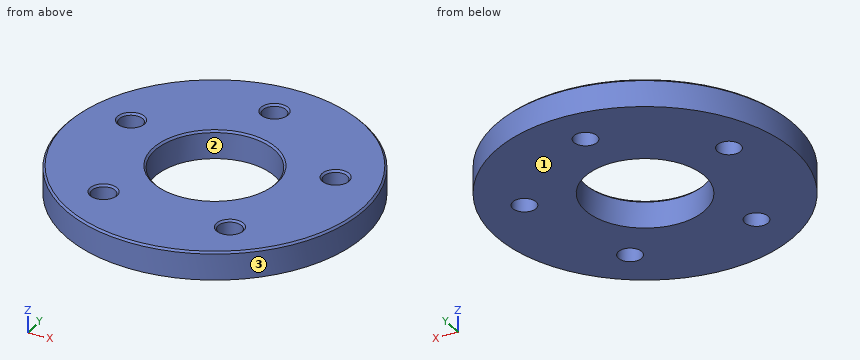
from build123d import *

# Parameters (mm, degrees)
F0_R     = 80
F0_R_2   = 6.25
F0_R_3   = 32.05
F1_DEPTH = 15
F2_SIZE  = 1


with BuildPart() as f1:
    # F0 (on Top) → F1 (new body)
    with BuildSketch(Plane.XY):
        Circle(F0_R)
        with Locations((-33.591927, -46.235321)):
            Circle(F0_R_2, mode=Mode.SUBTRACT)
        with Locations((33.591927, -46.235321)):
            Circle(F0_R_2, mode=Mode.SUBTRACT)
        with Locations((-54.35288, 17.660321)):
            Circle(F0_R_2, mode=Mode.SUBTRACT)
        Circle(F0_R_3, mode=Mode.SUBTRACT)
        with Locations((54.35288, 17.660321)):
            Circle(F0_R_2, mode=Mode.SUBTRACT)
        with Locations((0, 57.15)):
            Circle(F0_R_2, mode=Mode.SUBTRACT)
    extrude(amount=F1_DEPTH)

    # F2
    f2_edges = [f1.edges().sort_by_distance(p)[0] for p in [
        (-80, 0, 15),
        (-39.841927, -46.235321, 15),
        (27.341927, -46.235321, 15),
        (-60.60288, 17.660321, 15),
        (-32.05, 0, 15),
        (48.10288, 17.660321, 15),
        (-6.25, 57.15, 15),
    ]]
    chamfer(f2_edges, length=F2_SIZE)


solid = f1.part
Verification items for the finished model (mm, model axes). Face numbers are marked on the shaded views. Give positions to 0.01 mm unless a question says otherwise; leave off trailing zeros. Loops run counter-clockwise (first coordinate to the right, second up) from the corner with the lowest first, then second, coordinate; pieces in that order, holes last.
1) Sectioned sample at C-C, the plane z = 8.75. Enter the section's corners in (x, y), then the cut area to 3 significant figures.
2) Sectioned sample at B-B, the plane x = 0. Enter the section's corners in (y, z), then the cut area to 3 significant figures.
3) Thickness scan on line 1 along Y through (x, z) = (0, 4.5); line 2 along X through (y, z) = (0.5, 13.5); line 3 along X through (y, z) = (13.5, 12.5). Record the ranges inside material, lowest first.
4) Draft check along X on the marked faces 1, 2 and 3. Enter one of: pulls with the +X half, pulls with the -X half, needs draft (parallel to the pull), parting line crosses it, or undercut.
5) Depth check by flat-ended pin: pin 1 Ø3 at (y, z) = (6, 8) entering from +X; pin 2 Ø1 at (x, y) = (-44, 25) entering from -Z; pin 3 Ø2 at (y, z) = (26, 1.5) entering from +X; pin 4 Ø1.5 at (x, z) = (28.5, 5) entering from +Y. Enter the tip coordinate at first touch or a pass-through.
6) Sectioned sample at A-A, the plane y = 0. Enter the section's corners in (x, z).
Answers:
1. outline: circle Ø160 at (0, 0); hole circle Ø12.5 at (-54.35, 17.66); hole circle Ø12.5 at (-33.59, -46.24); hole circle Ø64.1 at (0, 0); hole circle Ø12.5 at (0, 57.15); hole circle Ø12.5 at (33.59, -46.24); hole circle Ø12.5 at (54.35, 17.66)
1. area: 16,300 mm2
2. outline: (-80, 0) - (-32.05, 0) - (-32.05, 14) - (-33.05, 15) - (-79, 15) - (-80, 14) - close; (32.05, 0) - (50.9, 0) - (50.9, 14) - (49.9, 15) - (33.05, 15) - (32.05, 14) - close; (63.4, 0) - (80, 0) - (80, 14) - (79, 15) - (64.4, 15) - (63.4, 14) - close
2. area: 1,250 mm2
3. line 1: y = -80 to -32.05, 32.05 to 50.9, 63.4 to 80
3. line 2: x = -80 to -32.05, 32.05 to 80
3. line 3: x = -78.85 to -59.02, -49.69 to -29.07, 29.07 to 49.69, 59.02 to 78.85
4. face 1: needs draft
4. face 2: undercut
4. face 3: parting line crosses it
5. pin 1: stops at x = 79.87
5. pin 2: stops at z = 0
5. pin 3: stops at x = 75.99
5. pin 4: stops at y = 75.03
6. outline: (-80, 0) - (-32.05, 0) - (-32.05, 14) - (-33.05, 15) - (-79, 15) - (-80, 14) - close; (32.05, 0) - (80, 0) - (80, 14) - (79, 15) - (33.05, 15) - (32.05, 14) - close
